CAD build for the part. Positions are in the model's coordinates, mm. Face numbers are marked on the shaded views. A direction names the side the tool comes from. Coordinates: 2 decimals unless noted, no trailing zeros. Order: outer loops, then holes, each group sorted by start corner. A loop starts at its lowest first (then second) coordinate and runs counter-clockwise, first axis right, second up. Notation, with made-up numbers: (-29.75, 56) - (-17.75, 56) arc R9 ccw to (-17.75, 61) - close; hole circle Ø9 at (-2.5, 16). An arc over 180 degrees is marked (long way). Use one line per item in the form item = value.
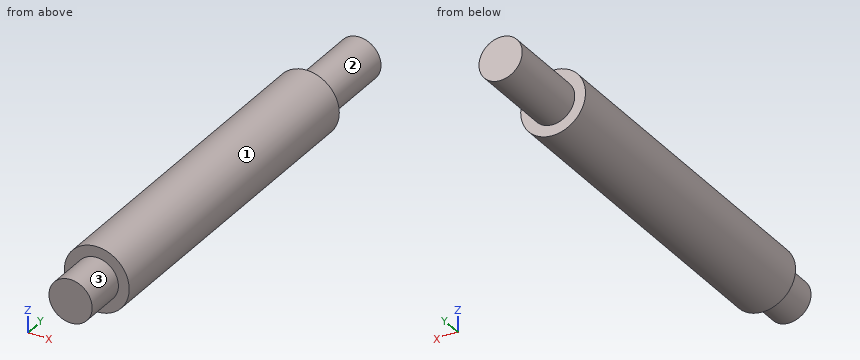
```python
from build123d import *

# Parameters (mm, degrees)
F0_R     = 9.525
F1_DEPTH = 101.6
F2_R     = 6.35
F3_DEPTH = 12.7
F4_R     = 6.35
F5_DEPTH = 25.4


with BuildPart() as f1:
    # F0 (on Front) → F1 (new body)
    with BuildSketch(Plane.XZ):
        Circle(F0_R)
    extrude(amount=F1_DEPTH)

    # F2 (on face) → F3 (join)
    with BuildSketch(Plane.XZ.offset(101.6)):
        Circle(F2_R)
    extrude(amount=F3_DEPTH)

    # F4 (on Front) → F5 (join)
    with BuildSketch(Plane.XZ):
        Circle(F4_R)
    extrude(amount=-F5_DEPTH)


solid = f1.part
```
Item 1: Drop flat-ended pins along their axis: pin 1 (3 mm diameter, centred on x = 2.5, y = -48.5, fed in from +Z); pin 2 (6 mm diameter, centred on y = 5.5, z = -5, fed in from +X); pin 3 (5 mm diameter, centred on x = 3, y = 6, fed in from -Z); pin 4 (5 mm diameter, centred on x = -7, z = -5, fed in from -Y). Give the stop position or say it passes through.
Derived:
pin_1 = 9.47
pin_2 = 6.03
pin_3 = -6.33
pin_4 = -114.3
Item 2: Cut at D-D, the plane y = -69.5. Write the cut outline in (x, z) (3 decimals).
Derived:
outline = circle Ø19.05 at (0, 0)
Item 3: Cut at B-B, the plane x = 0. Write the cut outline in (y, z) (3 decimals).
Derived:
outline = (-114.3, -6.35) - (-101.6, -6.35) - (-101.6, -9.525) - (0, -9.525) - (0, -6.35) - (25.4, -6.35) - (25.4, 6.35) - (0, 6.35) - (0, 9.525) - (-101.6, 9.525) - (-101.6, 6.35) - (-114.3, 6.35) - close
Item 4: Drill centre lines: line 1 (Y direction, x = -3, z = 7); line 2 (X direction, y = -68, z = 2); line 3 (X direction, y = -64, z = -7.5). Where is each one in solid material? Low to high. Write a range as [from, to].
Derived:
line_1 = [-101.6, 0]
line_2 = [-9.31, 9.31]
line_3 = [-5.87, 5.87]
Item 5: 3-axis set-ups, long thin cutter, end or side, ignore diameter. For the marked faces 1, 2 and 3: which of +Z, -Z, +X, -X, +Y, -Y reach the whole face in a straight line?
Derived:
face_1 = +Y, -Y
face_2 = +Y
face_3 = -Y
Item 6: Cut at A-A, the plane z = 0. Write the cut outline in (x, y) (3 decimals).
Derived:
outline = (-9.525, -101.6) - (-6.35, -101.6) - (-6.35, -114.3) - (6.35, -114.3) - (6.35, -101.6) - (9.525, -101.6) - (9.525, 0) - (6.35, 0) - (6.35, 25.4) - (-6.35, 25.4) - (-6.35, 0) - (-9.525, 0) - close
Item 7: Cut at C-C, the plane y = 10. Write the cut outline in (x, z), plus the area to 3 significant figures.
Derived:
outline = circle Ø12.7 at (0, 0)
area = 127 mm²
